The model under review builds one solid part; all positions refer to its coordinate system, in mm. Face numbers are marked on the shaded views. A direction names the side the tool comes from. Coordinates: 2 decimals unless noted, no trailing zeros. Order: outer loops, then holes, each group sorted by start corner. A loop starts at its lowest first (then second) coordinate and runs counter-clockwise, first axis right, second up.
Autodesk Inventor part; units mm, degrees
ref_plane "YZ Plane" through (0, 0, 0) normal (1, 0, 0) x (0, 1, 0)
ref_plane "XZ Plane" through (0, 0, 0) normal (0, 1, 0) x (-1, 0, 0)
ref_plane "XY Plane" through (0, 0, 0) normal (0, 0, 1) x (1, 0, 0)
sketch "Sketch1" plane through (0, 0, 0) normal (0, 0, 1) x (1, 0, 0)
  line L0 (127, 0) -> (127, 123.9012)
  line L1 (127, 123.9012) -> (0, 123.9012)
  line L2 (0, 123.9012) -> (0, 0)
  arc A0 (109.5375, 0) -> (68.2625, 0) centre (88.9, 0) ccw
  arc A1 (36.3964, 0) -> (14.4, 0) centre (25.3982, 0) ccw
  line L3 (14.4, 0) -> (0, 0)
  line L4 (127, 0) -> (109.5375, 0)
  line L5 (68.2625, 0) -> (36.3964, 0)
  dimension "d0" = 127
  dimension "d1" = 123.9012
  dimension "d2" = 41.275
  dimension "d25" = 38.1
  dimension "d26" = 21.9964
extrude "Extrusion1" add sketch "Sketch1" along normal blind 187.96
sketch "Sketch2" plane through (0, 123.9012, 0) normal (0, 1, 0) x (1, 0, 0)
  circle A0 centre (88.9, -152.4) radius 17.78
  line L0 (127, -187.96) -> (0, -187.96)
  line L1 (127, 0) -> (127, -187.96)
  circle A1 centre (88.9, -93.98) radius 17.78
  circle A2 centre (88.9, -35.56) radius 17.78
  line L2 (127, 0) -> (0, 0)
  point P0 (127, -35.56)
  point P1 (127, -93.98)
  point P2 (127, -152.4)
  dimension "d6" = 35.56
  dimension "d7" = 38.1
  dimension "d10" = 35.56
  dimension "d11" = 38.1
  dimension "d13" = 58.42
  dimension "d14" = 38.1
  dimension "d29" = 35.56
sketch "Sketch3" plane through (127, 0, 0) normal (1, 0, 0) x (0, 0, -1)
  line L0 (0, 123.9012) -> (-187.96, 123.9012)
  line L1 (0, 0) -> (-187.96, 0)
  line L2 (-35.56, 59.69) -> (-35.56, 0)
  line L3 (0, 0) -> (-187.96, 0)
  line L4 (-93.98, 0) -> (-93.98, 59.69)
  line L5 (-152.4, 59.69) -> (-152.4, 0)
  line L6 (0, 0) -> (0, 123.9012)
  line L7 (-187.96, 0) -> (-175.26, 0)
  line L8 (-175.26, 0) -> (-175.26, 59.69)
  line L9 (-175.26, 123.9012) -> (-187.96, 123.9012)
  line L10 (-187.96, 123.9012) -> (-187.96, 0)
  line L11 (-116.84, 0) -> (-129.54, 0)
  line L12 (-129.54, 0) -> (-129.54, 59.69)
  line L13 (-129.54, 123.9012) -> (-116.84, 123.9012)
  line L14 (-116.84, 59.69) -> (-116.84, 0)
  line L15 (-35.56, 59.69) -> (-35.56, 0)
  line L16 (0, 0) -> (-12.7, 0)
  line L17 (-12.7, 0) -> (-12.7, 59.69)
  line L18 (-12.7, 123.9012) -> (0, 123.9012)
  line L19 (0, 123.9012) -> (0, 0)
  line L20 (-71.12, 0) -> (-58.42, 0)
  line L21 (-58.42, 0) -> (-58.42, 59.69)
  line L22 (-58.42, 123.9012) -> (-71.12, 123.9012)
  line L23 (-71.12, 59.69) -> (-71.12, 0)
  line L24 (-187.96, 123.9012) -> (-187.96, 0)
  line L25 (-187.96, 123.9012) -> (0, 123.9012)
  line L26 (-58.42, 59.69) -> (-12.7, 59.69)
  line L27 (-175.26, 59.69) -> (-129.54, 59.69)
  line L28 (-116.84, 59.69) -> (-71.12, 59.69)
  dimension "d15" = 35.56
  dimension "d16" = 93.98
  dimension "d17" = 152.4
  dimension "d18" = 12.7
extrude "Extrusion2" cut sketch "Sketch3" against normal blind 187.96 contours L1 L2 L26 L17 | L1 L21 L26 L2 | L1 L4 L28 L23 | L1 L14 L28 L4 | L1 L5 L27 L12 | L8 L27 L5 L1
extrude "Extrusion3" cut sketch "Sketch2" against normal blind 187.96
sketch "Sketch4" plane through (127, 59.69, 129.54) normal (0, -1, 0) x (1, 0, 0)
  line L0 (-58.7375, -116.84) -> (-90.6036, -116.84)
  line L1 (-74.6705, -116.84) -> (-74.6705, 45.72)
  line L2 (-90.6036, 45.72) -> (-58.7375, 45.72)
  line L3 (-74.6705, 45.72) -> (-127, 45.72)
  line L4 (-127, -116.84) -> (-127, -71.12)
  line L5 (-127, 45.72) -> (-127, -116.84)
  line L6 (-127, -116.84) -> (-74.6705, -116.84)
  point P0 (-127, -129.54)
extrude "Extrusion4" add sketch "Sketch4" along normal blind 38.1
properties part number "E.Engine Block Top"
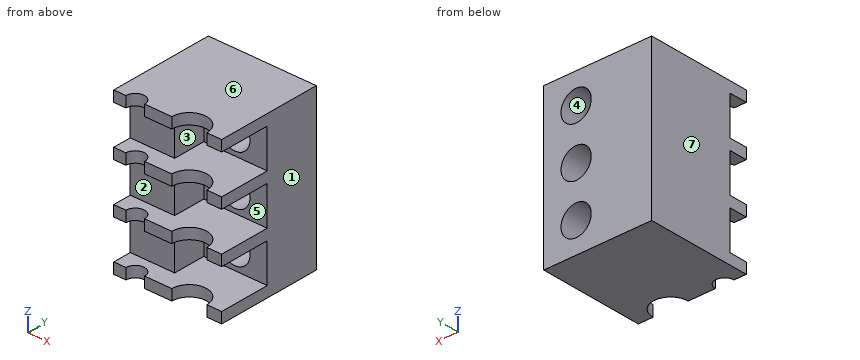
(1) We need section C-C, the plane x = 88.9. Write out the cut boundary in (y, z), and give its area (3 significant figures).
A:
outline: (20.64, 0) - (123.9, 0) - (123.9, 17.78) - (59.69, 17.78) - (59.69, 12.7) - (20.64, 12.7) - close; (20.64, 58.42) - (59.69, 58.42) - (59.69, 53.34) - (123.9, 53.34) - (123.9, 76.2) - (59.69, 76.2) - (59.69, 71.12) - (20.64, 71.12) - close; (20.64, 116.84) - (59.69, 116.84) - (59.69, 111.76) - (123.9, 111.76) - (123.9, 134.62) - (59.69, 134.62) - (59.69, 129.54) - (20.64, 129.54) - close; (20.64, 175.26) - (59.69, 175.26) - (59.69, 170.18) - (123.9, 170.18) - (123.9, 187.96) - (20.64, 187.96) - close
area: 7,200 mm2
(2) For pin 1 Ø5 at (x, z) = (25, 70) entering from -Y; pin 2 Ø10 at (y, z) = (12.5, 37.5) entering from +X; pin 3 Ø23 at (x, z) = (23, 149) entering from -Y; pin 4 Ø10 at (x, z) = (63, 148.5) entering from -Y, all flat-tipped, find the tip position at first contact; note any pin that passes through.
A:
pin 1: stops at y = 10.61
pin 2: passes through
pin 3: stops at y = 21.59
pin 4: stops at y = 59.69
(3) We need section A-A, the plane y = 88. Write out the cut boundary in (x, z), and give its area (3 significant figures).
A:
outline: (0, 0) - (127, 0) - (127, 187.96) - (0, 187.96) - close; hole circle Ø35.56 at (88.9, 35.56); hole circle Ø35.56 at (88.9, 93.98); hole circle Ø35.56 at (88.9, 152.4)
area: 20,900 mm2
(4) Machinability: for the marked faces 1, 2 and 3, which of the approach directions +Z, -Z, +X, -X, +Y, -Y give a long, thin tool a straight path to every point of the face, cutting with its end or side? Answer none if there is none.
A:
face 1: +Z, -Z, +X, +Y, -Y
face 2: +X, -X, -Y
face 3: +X, -Y
(5) We need section B-B, the plane z = 35.56. Write out the cut boundary in (x, y).
A:
outline: (0, 21.59) - (52.33, 21.59) - (52.33, 59.69) - (71.12, 59.69) - (71.12, 123.9) - (0, 123.9) - close; (106.68, 59.69) - (127, 59.69) - (127, 123.9) - (106.68, 123.9) - close
(6) We need section D-D, the plane x = 59. Write out the cut boundary in (y, z), and give its area (3 significant figures).
A:
outline: (0, 0) - (123.9, 0) - (123.9, 187.96) - (0, 187.96) - (0, 175.26) - (59.69, 175.26) - (59.69, 129.54) - (0, 129.54) - (0, 116.84) - (59.69, 116.84) - (59.69, 71.12) - (0, 71.12) - (0, 58.42) - (59.69, 58.42) - (59.69, 12.7) - (0, 12.7) - close
area: 15,100 mm2
(7) Wall thickness on probe 1 along Z at (x, y) = (88, 82); probe 2 along Z at (x, y) = (58.5, 49.5); probe 3 along X at (y, z) = (97, 93): over which ranges is each line inside the solid? List them lowest first.
A:
probe 1: z = 0 to 17.8, 53.32 to 76.22, 111.74 to 134.64, 170.16 to 187.96
probe 2: z = 0 to 12.7, 58.42 to 71.12, 116.84 to 129.54, 175.26 to 187.96
probe 3: x = 0 to 71.15, 106.65 to 127
(8) Draft analysis for pull direction Z (two halves, no side actions). For the marked faces 4, 5, 6 and 7, state which applies: released by +Z, released by -Z, zero draft, split by the parting line, or undercut.
A:
face 4: undercut
face 5: undercut
face 6: released by +Z
face 7: zero draft
